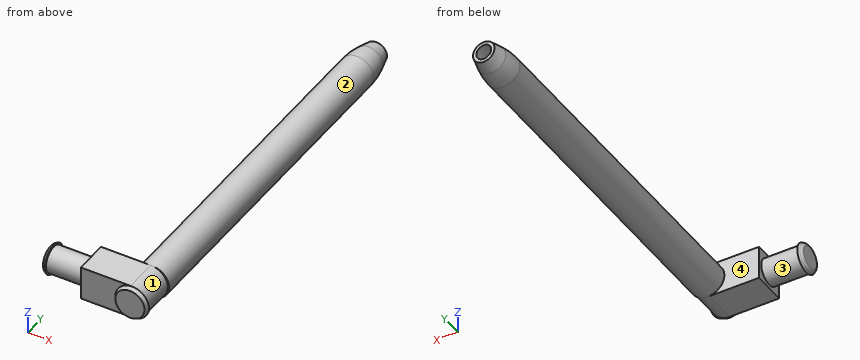
from build123d import *

# Parameters (mm, degrees)
SKETCH2_R           = 4.445
BOSS_EXTRUDE1_DEPTH = 6.35
SKETCH3_R           = 5.08
BOSS_EXTRUDE2_DEPTH = 1.27
BOSS_EXTRUDE2_TAPER = 30
FILLET1_R           = 1.27
SKETCH5_W           = 11.5062
SKETCH5_H           = 11.43
BOSS_EXTRUDE4_DEPTH = 22.86
CUT_EXTRUDE1_REACH  = 33.89
SKETCH6_R           = 2.54
FILLET2_R           = 5.842
SKETCH7_R           = 5.715
BOSS_EXTRUDE5_DEPTH = 1.27
BOSS_EXTRUDE5_TAPER = 30
BOSS_EXTRUDE6_START = 127
SKETCH8_R           = 5.715
SKETCH8_R_2         = 2.54
BOSS_EXTRUDE6_DEPTH = 127
CHAMFER1_SIZE       = 7.62
CHAMFER1_SIZE2      = 2.041772846
FILLET3_R           = 25.4


with BuildPart() as part:
    # Sketch2 → Boss-Extrude1 (new, symmetric)
    with BuildSketch(Plane(origin=(0, 0, 0), x_dir=(0, 0, -1), z_dir=(1, 0, 0))):
        with Locations(Location((0, 0, 0), (0, 0, 180))):
            Circle(SKETCH2_R)
    extrude(amount=BOSS_EXTRUDE1_DEPTH, both=True)

    # Sketch3 → Boss-Extrude2 (add)
    with BuildSketch(Plane.ZY.offset(6.35)):
        Circle(SKETCH3_R)
    extrude(amount=BOSS_EXTRUDE2_DEPTH, taper=BOSS_EXTRUDE2_TAPER)

    # Fillet1
    fillet1_edges = [part.edges().sort_by_distance(p)[0] for p in [
        (-7.62, 0, -4.346765158),
    ]]
    fillet(fillet1_edges, radius=FILLET1_R)

    # Sketch5 → Boss-Extrude4 (add)
    with BuildSketch(Plane(origin=(6.35, 0, 0), x_dir=(0, 0, -1), z_dir=(1, 0, 0))):
        Rectangle(SKETCH5_W, SKETCH5_H)
    extrude(amount=BOSS_EXTRUDE4_DEPTH)

    # Sketch6 → Cut-Extrude1 (cut, up to next)
    with BuildSketch(Plane(origin=(0, 5.715, 0), x_dir=(1, 0, 0), z_dir=(0, 1, 0)), mode=Mode.PRIVATE) as cut_extrude1_sk1:
        with Locations(Location((23.876, 0, 0), (0, 0, 270))):
            Circle(SKETCH6_R)
    cut_extrude1_tool1 = extrude(cut_extrude1_sk1.sketch, amount=-CUT_EXTRUDE1_REACH, mode=Mode.PRIVATE) & part.part
    add(cut_extrude1_tool1.solids().sort_by_distance((23.876, 5.715, 0))[0], mode=Mode.SUBTRACT)

    # Fillet2
    # the kernel refuses this fillet: 5.842 mm, written as the material it takes off along each edge
    with BuildSketch(Plane(origin=(29.21, -20.32, -5.7531), x_dir=(0, 0, 1), z_dir=(0, 1, 0))) as fillet2_piece_1:
        with BuildLine():
            CenterArc((FILLET2_R, -FILLET2_R), FILLET2_R, 90, 90)
            Line((0, -FILLET2_R), (0, 0))
            Line((0, 0), (FILLET2_R, 0))
        make_face()
    extrude(amount=40.64, mode=Mode.SUBTRACT)
    with BuildSketch(Plane(origin=(29.21, 20.32, 5.7531), x_dir=(-1, 0, 0), z_dir=(0, -1, 0))) as fillet2_piece_2:
        with BuildLine():
            CenterArc((FILLET2_R, FILLET2_R), FILLET2_R, 180, 90)
            Line((0, FILLET2_R), (0, 0))
            Line((0, 0), (FILLET2_R, 0))
        make_face()
    extrude(amount=40.64, mode=Mode.SUBTRACT)

    # Sketch7 → Boss-Extrude5 (add)
    with BuildSketch(Plane.XZ.offset(5.715)):
        with Locations((23.876, 0)):
            Circle(SKETCH7_R)
    extrude(amount=BOSS_EXTRUDE5_DEPTH, taper=BOSS_EXTRUDE5_TAPER)

    # Sketch8 → Boss-Extrude6 (add)
    with BuildSketch(Plane(origin=(0, 5.715, 0), x_dir=(1, 0, 0), z_dir=(0, 1, 0)).offset(BOSS_EXTRUDE6_START)):
        with Locations(Location((23.876, 0, 0), (0, 0, 88.162656718))):
            Circle(SKETCH8_R)
        with Locations(Location((23.876, 0, 0), (0, 0, 270))):
            Circle(SKETCH8_R_2, mode=Mode.SUBTRACT)
    extrude(amount=-BOSS_EXTRUDE6_DEPTH)

    # Chamfer1
    chamfer1_edges = [part.edges().sort_by_distance(p)[0] for p in [
        (23.692764561, 132.715, 5.71206178),
    ]]
    chamfer1_side = [part.faces().sort_by_distance(p)[0] for p in [
        (23.692764561, 69.215, 5.71206178),
    ]]
    chamfer(chamfer1_edges, length=CHAMFER1_SIZE, length2=CHAMFER1_SIZE2, reference=chamfer1_side[0])

    # Fillet3
    fillet3_edges = [part.edges().sort_by_distance(p)[0] for p in [
        (23.692764561, 125.095, 5.71206178),
    ]]
    fillet(fillet3_edges, radius=FILLET3_R)


solid = part.part
Input: part model. Units: mm. Frame: model coordinates. Face numbers are marked on the shaded views. Coordinates: 2 decimals unless noted, no trailing zeros. Loops run counter-clockwise (first coordinate to the right, second up) from the corner with the lowest first, then second, coordinate; pieces in that order, holes last.
Q1. Contact query for flat-ended pins moving along their axis: pin 1 (1 mm diameter, centred on x = 24, y = 43, fed in from -Z) (3 decimals); pin 2 (5 mm diameter, centred on y = 76.5, z = -1, fed in from -X); pin 3 (4 mm diameter, centred on x = 19.5, y = 112.5, fed in from -Z). Output: stop coordinate, or through.
Q2. Draft query along Y for the marked faces 1, 2, 3 and 4. Return one class per face: +Y half, -Y half, draft (parallel to the pull), parting line (faces both ways), or undercut.
Q3. Cut plane A-A (y = 74). Output: boundary loops of the cut face in (x, z) (3 decimals), then the cut area to 3 significant figures.
Q4. Material intervals for line 1 (X direction, y = 59.5, z = 0); line 2 (Z direction, x = 24, y = 25.5); line 3 (Z direction, x = 26.5, y = 3), sorted ascending.
Working result:
1. pin 1: stops at z = -5.715
1. pin 2: stops at x = 18.16
1. pin 3: stops at z = -5.2
2. face 1: undercut
2. face 2: draft
2. face 3: parting line
2. face 4: +Y half
3. outline: circle Ø11.43 at (23.876, 0); hole circle Ø5.08 at (23.876, 0)
3. area: 82.3 mm2
4. line 1: x = 18.16 to 21.34, 26.42 to 29.59
4. line 2: z = -5.71 to -2.54, 2.54 to 5.71
4. line 3: z = -4.84 to 4.84
